Could you check a few things on this model? Use its own coordinates, in mm. Face numbers are marked on the shaded views. Coordinates: 2 decimals unless noted, no trailing zeros. Write each loop counter-clockwise with the first axis right and the second up, starting at its lowest first coordinate (ties: lowest second). Pieces come first, ordered by that corner, then holes. Notation, with made-up numbers: (-37, 60) - (15, 60) arc R31 cw to (15, 98) - close; hole circle Ø5 at (44, -29). An arc over 180 degrees is marked (long way). Answer as a JSON object with one key per item and string values. Group by question number.
1) If we section it at A-A (x = 0): Write out the boundary of the cut face in (y, z), plus the area to 3 significant figures.
2) If we section it at D-D (y = 4.25): Write out the boundary of the cut face in (x, z).
3) Will these pins go through, and if not, where does the flat tip stop? pin 1 Ø4 at (y, z) = (6.5, 19.5) entering from -X; pin 2 Ø1.5 at (y, z) = (7, -21.5) entering from -X; pin 3 Ø4 at (x, y) = (-16, 1) entering from -Z.
4) If we section it at C-C (x = 16): Write out the boundary of the cut face in (y, z), plus the area to 3 significant figures.
5) Please list where these lines run through material, in increasing order: line 1 along Z through (x, y) = (0, 4); line 2 along Z through (x, y) = (3, 0.5); line 3 along Z through (x, y) = (13, -0.25).
6) If we section it at B-B (z = 0): Write out the boundary of the cut face in (x, y).
7) We'd pull the mould along X, two halves only. Please class the marked faces 1, 2 and 3: released by +X, released by -X, zero draft, split by the parting line, or undercut.
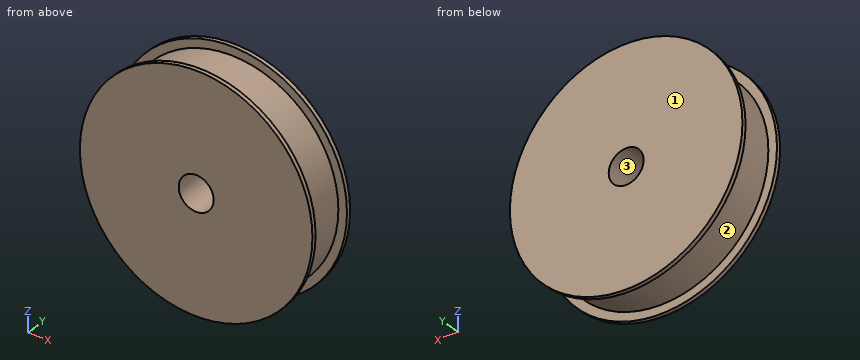
Autodesk Inventor part; units mm, degrees
ref_plane "YZ Plane" through (0, 0, 0) normal (1, 0, 0) x (0, 1, 0)
ref_plane "XZ Plane" through (0, 0, 0) normal (0, 1, 0) x (-1, 0, 0)
ref_plane "XY Plane" through (0, 0, 0) normal (0, 0, 1) x (1, 0, 0)
sketch "スケッチ1" plane through (0, 0, 0) normal (0, 1, 0) x (-1, 0, 0)
  circle A0 centre (0, 0) radius 25
  dimension "d0" = 50
extrude "押し出し1" add sketch "スケッチ1" along normal blind 10
sketch "スケッチ2" plane through (0, 10, 0) normal (0, 1, 0) x (1, 0, 0)
  circle A0 centre (0, 0) radius 27
  dimension "d3" = 54
extrude "押し出し2" add sketch "スケッチ2" along normal blind 1
sketch "スケッチ3" plane through (0, 0, 0) normal (0, -1, 0) x (1, 0, 0)
  circle A0 centre (0, 0) radius 27
  dimension "d6" = 54
extrude "押し出し3" add sketch "スケッチ3" along normal blind 1
sketch "スケッチ4" plane through (0, 11, 0) normal (0, 1, 0) x (1, 0, 0)
  circle A0 centre (0, 0) radius 4.05
  dimension "d9" = 8.1
extrude "押し出し4" cut sketch "スケッチ4" against normal blind 12
properties part number "NHK"
Here are the results:
{
 "1": {"outline": "(-1, -27) - (0, -27) - (0, -25) - (10, -25) - (10, -27) - (11, -27) - (11, -4.05) - (-1, -4.05) - close; (-1, 4.05) - (11, 4.05) - (11, 27) - (10, 27) - (10, 25) - (0, 25) - (0, 27) - (-1, 27) - close", "area": "511 mm²"},
 "2": {"outline": "circle Ø50 at (0, 0); hole circle Ø8.1 at (0, 0)"},
 "3": {"pin 1": "stops at x = -17.85", "pin 2": "stops at x = -13.94", "pin 3": "stops at z = -22.92"},
 "4": {"outline": "(-1, -21.75) - (0, -21.75) - (0, -19.21) - (10, -19.21) - (10, -21.75) - (11, -21.75) - (11, 21.75) - (10, 21.75) - (10, 19.21) - (0, 19.21) - (0, 21.75) - (-1, 21.75) - close", "area": "471 mm²"},
 "5": {"line 1": "z = -25 to -4.05, 4.05 to 25", "line 2": "z = -24.82 to -2.72, 2.72 to 24.82", "line 3": "z = -23.66 to 23.66"},
 "6": {"outline": "(-27, -1) - (-4.05, -1) - (-4.05, 11) - (-27, 11) - (-27, 10) - (-25, 10) - (-25, 0) - (-27, 0) - close; (4.05, -1) - (27, -1) - (27, 0) - (25, 0) - (25, 10) - (27, 10) - (27, 11) - (4.05, 11) - close"},
 "7": {"face 1": "zero draft", "face 2": "split by the parting line", "face 3": "undercut"}
}
